Verification items for the finished model (mm, model axes). A direction names the side the tool comes from. Round coordinates to 2 decimals unless told otherwise and drop trailing zeros. Write each loop counter-clockwise with the first axis right and the second up, starting at its lowest first coordinate (ties: lowest second). Pieces come first, ordered by that corner, then holes. Notation, with made-up numbers: M 72,45 L 129,45 A21 ccw 129,80 Z; hole C 38,-11.75 d10. An arc over 180 degrees is marked long. One line per question, with ' | ' between items.
from build123d import *

# Parameters (mm, degrees)
CROQUIS1_R              = 1.35
CROQUIS1_R_2            = 4
CROQUIS1_R_3            = 1.25
SALIENTE_EXTRUIR1_DEPTH = 4
REDONDEO1_R             = 1.6
CROQUIS2_R              = 1
CROQUIS2_R_2            = 3
CORTAR_EXTRUIR1_DEPTH   = 4


with BuildPart() as part:
    # Croquis1 → Saliente-Extruir1 (new body)
    with BuildSketch(Plane.XY):
        with BuildLine():
            Line((-15, -10.656453444), (-15, -73.656453444))
            Line((-15, -73.656453444), (15, -73.656453444))
            Line((15, -73.656453444), (15, -10.656453444))
            ThreePointArc((15, -10.656453444), (0, 18.4), (-15, -10.656453444))
        make_face()
        with Locations((-7.071067812, -7.071067812)):
            Circle(CROQUIS1_R, mode=Mode.SUBTRACT)
        with Locations((-7.071067812, 7.071067812)):
            Circle(CROQUIS1_R, mode=Mode.SUBTRACT)
        with Locations((7.071067812, 7.071067812)):
            Circle(CROQUIS1_R, mode=Mode.SUBTRACT)
        with Locations((7.071067812, -7.071067812)):
            Circle(CROQUIS1_R, mode=Mode.SUBTRACT)
        Circle(CROQUIS1_R_2, mode=Mode.SUBTRACT)
        with Locations((-10, -70.656453444)):
            Circle(CROQUIS1_R, mode=Mode.SUBTRACT)
        with Locations(Location((10, -70.656453444, 0), (0, 0, 180))):
            Circle(CROQUIS1_R, mode=Mode.SUBTRACT)
        with Locations((9.5, -54.791192074)):
            Circle(CROQUIS1_R_3, mode=Mode.SUBTRACT)
        with Locations((-9.5, -31.791192074)):
            Circle(CROQUIS1_R_3, mode=Mode.SUBTRACT)
    extrude(amount=SALIENTE_EXTRUIR1_DEPTH)

    # Redondeo1
    redondeo1_edges = [part.edges().sort_by_distance(p)[0] for p in [
        (15, -10.656453444, 2),
        (15, -73.656453444, 2),
        (-15, -73.656453444, 2),
        (-15, -10.656453444, 2),
    ]]
    fillet(redondeo1_edges, radius=REDONDEO1_R)

    # Croquis2 → Cortar-Extruir1 (cut)
    with BuildSketch(Plane.XY.offset(4)):
        with Locations((0, -52.656453444)):
            Circle(CROQUIS2_R)
        with Locations((-9, -63.656453444)):
            Circle(CROQUIS2_R_2)
    extrude(amount=-CORTAR_EXTRUIR1_DEPTH, mode=Mode.SUBTRACT)


solid = part.part
1. Section check A-A, the plane y = 0. Record the cut outline in (x, z), then the cut area to 3 significant figures.
Results:
outline: M -18.4,0 L -4,0 L -4,4 L -18.4,4 Z; M 4,0 L 18.4,0 L 18.4,4 L 4,4 Z | area: 115 mm2
2. Section check C-C, the plane x = 9.5. Record the cut outline in (y, z).
Results:
outline: M -73.66,0 L -71.91,0 L -71.91,4 L -73.66,4 Z; M -69.4,0 L -56.04,0 L -56.04,4 L -69.4,4 Z; M -53.54,0 L 15.76,0 L 15.76,4 L -53.54,4 Z
3. Section check D-D, the plane z = 1.05. Count the separate pieces of the cut face and the enclosed holes in it, then the cut area to 3 significant figures.
Results:
separate pieces: 1 | enclosed holes: 11 | area: 2,660 mm2
4. Go/stop test with a flat-tipped pin: P1, Ø1.5, axis at y = -58.5, z = 2.5, coming from the -X side. Record where the tip stops, or that it passes through.
Results:
P1: stops at x = -15
5. Section check B-B, the plane x = -9.5. Record the cut outline in (y, z).
Results:
outline: M -73.66,0 L -71.91,0 L -71.91,4 L -73.66,4 Z; M -69.4,0 L -66.61,0 L -66.61,4 L -69.4,4 Z; M -60.7,0 L -33.04,0 L -33.04,4 L -60.7,4 Z; M -30.54,0 L 15.76,0 L 15.76,4 L -30.54,4 Z
6. Tool access check on faces 1 (the face through (15, -42, 2)), 2 (the face through (-15, -41, 2)), 3 (the face through (0, -27, 0)). Record the directions out of +Z, -Z, +X, -X, +Y, -Y that give a thin tool (end or side, any length) a straight path to the whole face; none if there is none.
Results:
face 1: +Z, -Z, +X, -Y | face 2: +Z, -Z, -X, -Y | face 3: -Z, +X, -X, +Y, -Y
7. Thickness scan on line 1 (Y direction, x = 9.5, z = 1.8); line 2 (Y direction, x = -10.5, z = 1); line 3 (Y direction, x = 0, z = 3.2). Record the ranges inside material, lowest first.
Results:
line 1: y = -73.66 to -71.91, -69.4 to -56.04, -53.54 to 15.76 | line 2: y = -73.66 to -71.91, -69.4 to -66.25, -61.06 to -32.54, -31.04 to 15.11 | line 3: y = -73.66 to -53.66, -51.66 to -4, 4 to 18.4
8. Mould release check, pull along Y, two halves, no side actions. Record for faces 4 (the face through (14.52, -73.2, 2.03)), 5 (the face through (0.56, 18.39, 1.97)), 6 (the face through (-9.39, -60.68, 2.03)): pulls with the +Y half, pulls with the -Y half, needs draft (parallel to the pull), parting line crosses it, or undercut.
Results:
face 4: pulls with the -Y half | face 5: parting line crosses it | face 6: undercut
